Here's the drawing with two shaded views (mm, measured from the low corner). I have some questions. A direction names the side the tool comes from. Coordinates: 2 decimals unless noted, no trailing zeros. Loops run counter-clockwise (first coordinate to the right, second up) from the corner with the lowest first, then second, coordinate; pieces in that order, holes last. Notation, with made-up numbers: (54, 71) -> (82, 71) arc R20 ccw to (82, 82) -> close; hole circle Ø11 at (5.5, 56). An arc over 180 degrees is marked (long way). Answer as a JSON object with one key per item and string values. Group by question number.
1) I want a section at A-A (y = 4.25). Write out the boundary of the cut face in (x, z).
2) Which directions (+Z, -Z, +X, -X, +Y, -Y) give clear straight access to the entire face, cutting with the end or side of a thin tool? Please do the marked faces 1 and 2.
3) I want a section at D-D (z = 6.75). Write out the boundary of the cut face in (x, y).
4) I want a section at C-C (z = 3). Write out the boundary of the cut face in (x, y), then the cut area to 3 significant figures.
5) I'm going to push a flat-ended pin straight in: pin 1 (1 mm diameter, centred on x = 6.5, z = 3, fed in from +Y). Where does the tip first touch, or does it pass through?
6) I need wall thicknesses on probe 1 along Z at (x, y) = (5, 1); probe 2 along Y at (x, z) = (4.25, 0.75); probe 3 along Y at (x, z) = (5, 4). Which ranges of each line are inside material? Lowest first, please. Write a range as [from, to].
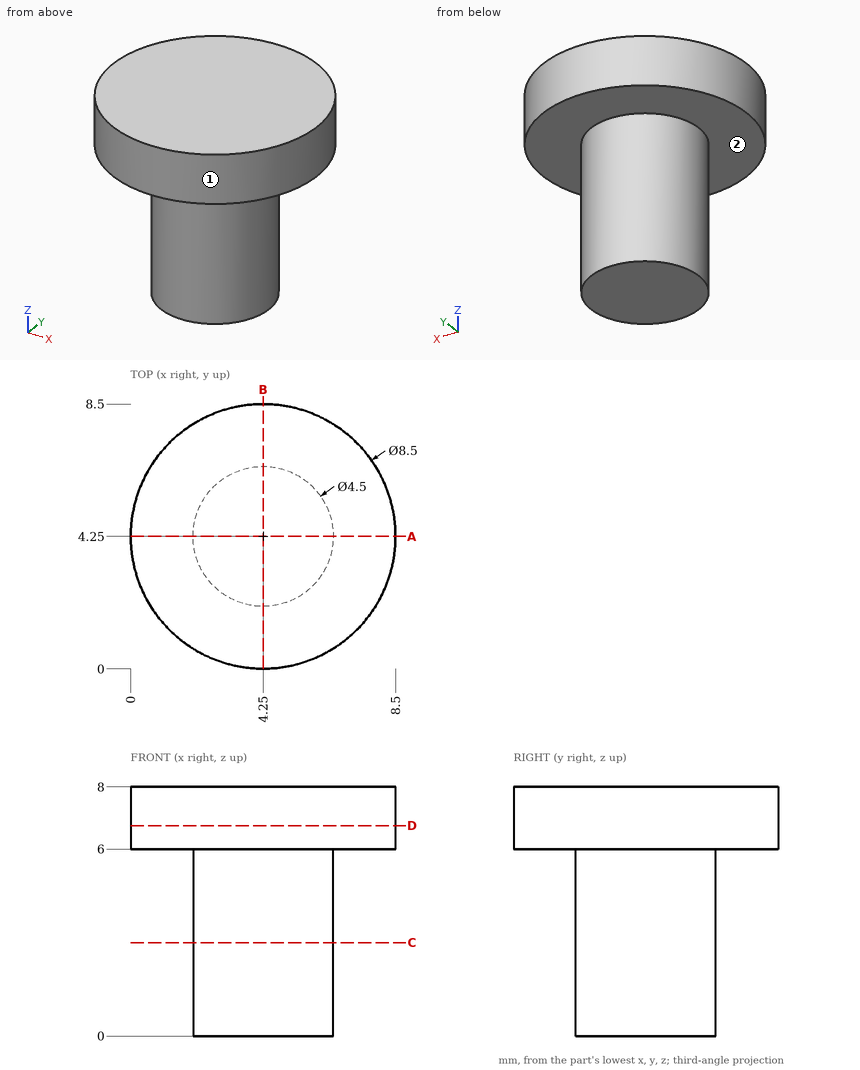
Determined:
{
 "1": {"outline": "(0, 6) -> (2, 6) -> (2, 0) -> (6.5, 0) -> (6.5, 6) -> (8.5, 6) -> (8.5, 8) -> (0, 8) -> close"},
 "2": {"face 1": "+Z, -Z", "face 2": "-Z"},
 "3": {"outline": "circle Ø8.5 at (4.25, 4.25)"},
 "4": {"outline": "circle Ø4.5 at (4.25, 4.25)", "area": "15.9 mm^2"},
 "5": {"pin 1": "y = 5.66"},
 "6": {"probe 1": "[6, 8]", "probe 2": "[2, 6.5]", "probe 3": "[2.13, 6.37]"}
}
